```python
from build123d import *

# Parameters (mm, degrees)
SKETCH1_W                = 80
SKETCH1_H                = 140
SKETCH1_R                = 2.5
BOSS_EXTRUDE1_DEPTH      = 6.35
SKETCH3_W                = 140
SKETCH3_H                = 179.9
BOSS_EXTRUDE2_DEPTH      = 6.35
BOSS_EXTRUDE3_DEPTH      = 70
BOSS_EXTRUDE3_DEPTH_BACK = 70
CUT_EXTRUDE1_DEPTH       = 63.65
CUT_EXTRUDE1_DEPTH_BACK  = 63.65


with BuildPart() as part:
    # Sketch1 → Boss-Extrude1 (new body)
    with BuildSketch(Plane(origin=(0, 0, 0), x_dir=(1, 0, 0), z_dir=(0, 1, 0))):
        with Locations((40, 0)):
            Rectangle(SKETCH1_W, SKETCH1_H)
        with Locations(Location((5, 0, 0), (0, 0, 270))):
            Circle(SKETCH1_R, mode=Mode.SUBTRACT)
        with BuildLine():
            Line((12.5, 24.05), (27.5, 24.05))
            ThreePointArc((27.5, 24.05), (31.55, 20), (27.5, 15.95))
            Line((27.5, 15.95), (12.5, 15.95))
            ThreePointArc((12.5, 15.95), (8.45, 20), (12.5, 24.05))
        make_face(mode=Mode.SUBTRACT)
        with BuildLine():
            Line((52.5, 24.05), (67.5, 24.05))
            ThreePointArc((67.5, 24.05), (71.55, 20), (67.5, 15.95))
            Line((67.5, 15.95), (52.5, 15.95))
            ThreePointArc((52.5, 15.95), (48.45, 20), (52.5, 24.05))
        make_face(mode=Mode.SUBTRACT)
        with BuildLine():
            Line((52.5, -15.95), (67.5, -15.95))
            ThreePointArc((67.5, -15.95), (71.55, -20), (67.5, -24.05))
            Line((67.5, -24.05), (52.5, -24.05))
            ThreePointArc((52.5, -24.05), (48.45, -20), (52.5, -15.95))
        make_face(mode=Mode.SUBTRACT)
        with BuildLine():
            Line((12.5, -15.95), (27.5, -15.95))
            ThreePointArc((27.5, -15.95), (31.55, -20), (27.5, -24.05))
            Line((27.5, -24.05), (12.5, -24.05))
            ThreePointArc((12.5, -24.05), (8.45, -20), (12.5, -15.95))
        make_face(mode=Mode.SUBTRACT)
    extrude(amount=-BOSS_EXTRUDE1_DEPTH)

    # Sketch3 → Boss-Extrude2 (add)
    with BuildSketch(Plane(origin=(0, 0, 0), x_dir=(0, 0, -1), z_dir=(1, 0, 0))):
        with Locations((0, 89.95)):
            Rectangle(SKETCH3_W, SKETCH3_H)
        with BuildLine():
            Line((-40.45, 169.45), (-40.45, 154.45))
            ThreePointArc((-40.45, 154.45), (-44.5, 150.4), (-48.55, 154.45))
            Line((-48.55, 154.45), (-48.55, 169.45))
            ThreePointArc((-48.55, 169.45), (-44.5, 173.5), (-40.45, 169.45))
        make_face(mode=Mode.SUBTRACT)
        with BuildLine():
            Line((48.55, 169.45), (48.55, 154.45))
            ThreePointArc((48.55, 154.45), (44.5, 150.4), (40.45, 154.45))
            Line((40.45, 154.45), (40.45, 169.45))
            ThreePointArc((40.45, 169.45), (44.5, 173.5), (48.55, 169.45))
        make_face(mode=Mode.SUBTRACT)
        with BuildLine():
            Line((48.55, 80.45), (48.55, 65.45))
            ThreePointArc((48.55, 65.45), (44.5, 61.4), (40.45, 65.45))
            Line((40.45, 65.45), (40.45, 80.45))
            ThreePointArc((40.45, 80.45), (44.5, 84.5), (48.55, 80.45))
        make_face(mode=Mode.SUBTRACT)
        with BuildLine():
            Line((-40.45, 80.45), (-40.45, 65.45))
            ThreePointArc((-40.45, 65.45), (-44.5, 61.4), (-48.55, 65.45))
            Line((-48.55, 65.45), (-48.55, 80.45))
            ThreePointArc((-48.55, 80.45), (-44.5, 84.5), (-40.45, 80.45))
        make_face(mode=Mode.SUBTRACT)
        with BuildLine():
            Line((30, 124.95), (30, 109.95))
            ThreePointArc((30, 109.95), (0, 79.95), (-30, 109.95))
            Line((-30, 109.95), (-30, 124.95))
            ThreePointArc((-30, 124.95), (0, 154.95), (30, 124.95))
        make_face(mode=Mode.SUBTRACT)
    extrude(amount=BOSS_EXTRUDE2_DEPTH)

    # Sketch4 → Boss-Extrude3 (add, two sides: drawn at the far end of the back side and taken through both)
    with BuildSketch(Plane.XY.offset(-BOSS_EXTRUDE3_DEPTH_BACK)):
        Polygon((6.35, 179.9), (80, 0), (6.35, 0), align=None)
    extrude(amount=BOSS_EXTRUDE3_DEPTH + BOSS_EXTRUDE3_DEPTH_BACK)

    # Sketch5 → Cut-Extrude1 (cut, two sides: drawn at the far end of the back side and taken through both)
    with BuildSketch(Plane.XY.offset(-CUT_EXTRUDE1_DEPTH_BACK)):
        Polygon((6.35, 179.9), (80, 0), (6.35, 0), align=None)
    extrude(amount=CUT_EXTRUDE1_DEPTH + CUT_EXTRUDE1_DEPTH_BACK, mode=Mode.SUBTRACT)


solid = part.part
```
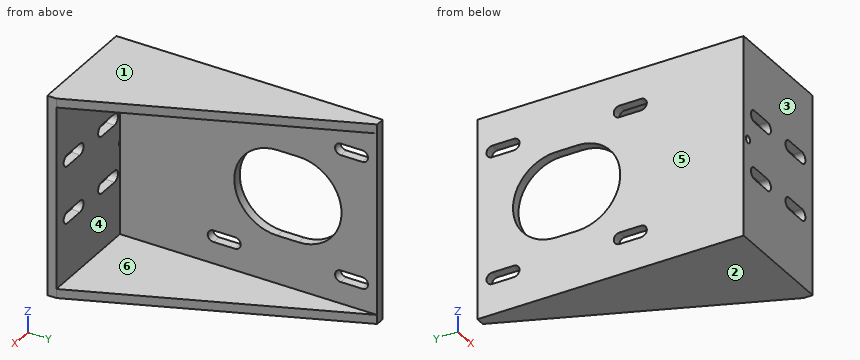
Input: part model. Units: mm. Frame: model coordinates. Face numbers are marked on the shaded views. A direction names the side the tool comes from. Coordinates: 2 decimals unless noted, no trailing zeros. Order: outer loops, then holes, each group sorted by start corner. A loop starts at its lowest first (then second) coordinate and runs counter-clockwise, first axis right, second up. Notation, with made-up numbers: (52.25, 25) - (108.25, 25) arc R21 cw to (108.25, 44) - close; hole circle Ø1 at (11, -26). An arc over 180 degrees is marked (long way). Return JSON: item names as keys, results as strings.
Q1. Cut plane A-A (z = 46). Return loops of the section in (x, y), then the cut area to 3 significant figures.
The answers:
{"outline": "(0, -6.35) - (80, -6.35) - (80, 0) - (6.35, 0) - (6.35, 61.69) - (0, 61.69) - close; (0, 84.21) - (6.35, 84.21) - (6.35, 150.69) - (0, 150.69) - close; (0, 173.21) - (6.35, 173.21) - (6.35, 179.9) - (0, 179.9) - close", "area": "1,360 mm2"}
Q2. Cut plane C-C (z = -6). Return loops of the section in (x, y), then the cut area to 3 significant figures.
The answers:
{"outline": "(0, -6.35) - (80, -6.35) - (80, 0) - (6.35, 0) - (6.35, 80.56) - (0, 80.56) - close; (0, 154.34) - (6.35, 154.34) - (6.35, 179.9) - (0, 179.9) - close", "area": "1,180 mm2"}
Q3. Cut plane B-B (y = 163). Return loops of the section in (x, z), then the cut area to 3 significant figures.
The answers:
{"outline": "(0, -70) - (13.27, -70) - (13.27, -63.65) - (6.35, -63.65) - (6.35, -48.55) - (0, -48.55) - close; (0, -40.45) - (6.35, -40.45) - (6.35, 40.45) - (0, 40.45) - close; (0, 48.55) - (6.35, 48.55) - (6.35, 63.65) - (13.27, 63.65) - (13.27, 70) - (0, 70) - close", "area": "874 mm2"}
Q4. Access query for the marked faces 5 and 6. Directions: +Z, -Z, +X, -X, +Y, -Y. A direction counts if a zero-diameter tool reaches every point of the face in a straight line with its end or side. Return the directions, or none.
The answers:
{"face 5": "+Z, -Z, -X, +Y, -Y", "face 6": "+X, +Y"}
Q5. Cut plane D-D (x = 64.5). Return loops of the section in (y, z).
The answers:
{"outline": "(-6.35, -70) - (37.86, -70) - (37.86, -63.65) - (0, -63.65) - (0, -24.05) - (-6.35, -24.05) - close; (-6.35, -15.95) - (0, -15.95) - (0, 15.95) - (-6.35, 15.95) - close; (-6.35, 24.05) - (0, 24.05) - (0, 63.65) - (37.86, 63.65) - (37.86, 70) - (-6.35, 70) - close"}
Q6. Draft query along Z for the marked faces 1, 2, 3 and 4. Return one class per face: +Z half, -Z half, draft (parallel to the pull), parting line (faces both ways), or undercut.
The answers:
{"face 1": "+Z half", "face 2": "-Z half", "face 3": "draft", "face 4": "undercut"}
Q7. First-contact query: pin 1 (10 mm diameter, centred on y = 28.5, z = -39, fed in from +X); pin 2 (12 mm diameter, centred on x = 36.5, z = -31.5, fed in from +Y). Flat tips, straight axial feed; report the tip coordinate or a pass-through.
The answers:
{"pin 1": "stops at x = 6.35", "pin 2": "stops at y = 0"}
Q8. Ray query, probe 1 along Z at (x, y) = (52, 27.5); probe 2 along X at (y, z) = (-4.5, 0); probe 3 along Z at (x, y) = (5, -3.75). Return the intervals inside material, ascending.
The answers:
{"probe 1": "z = -70 to -63.65, 63.65 to 70", "probe 2": "x = 0 to 2.5, 7.5 to 80", "probe 3": "z = -70 to -2.5, 2.5 to 70"}
